Check sheet for the drawn part. Datum: minimum x, y, z corner. Units: mm. A direction names the side the tool comes from. Round coordinates to 2 decimals unless told otherwise and drop trailing zeros. Order: outer loops, then holes, each group sorted by start corner. A loop starts at its lowest first (then second) coordinate and runs counter-clockwise, first axis right, second up. Notation, with made-up numbers: (78.25, 35) -> (83.25, 35) arc R33 cw to (83.25, 69) -> close; hole circle Ø6 at (40.5, 19). An arc over 180 degrees is marked (long way). Write item = value, one per line. Start each with the question number.
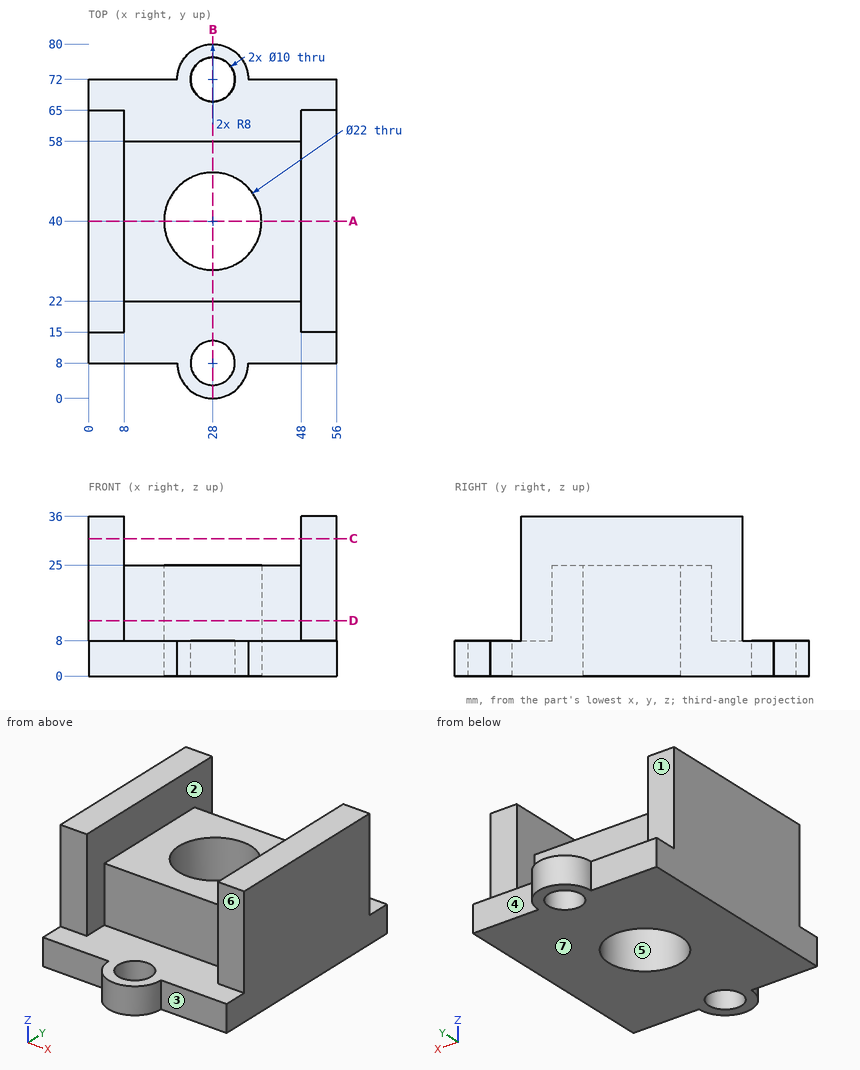
(1) Cross-section at B-B (x = 28). Enter the section's corners in (y, z), and give its area (3 significant figures).
(2) Depth check by flat-ended pin: pin 1 (9 mm diameter, centred on x = 51, z = 5.5, fed in from +Y); pin 2 (4 mm diameter, centred on x = 50, z = 25, fed in from +Y); pin 3 (14 mm diameter, centred on y = 39.5, z = 19, fed in from -X); pin 4 (1 mm diameter, centred on x = 16, y = 65, fed in from +Z). Enter the tip coordinate at first touch or a pass-through.
(3) Set-up check for the marked faces 1, 2, 3 and 4: record each of +Z, -Z, +X, -X, +Y, -Y from which the full face is reachable in a straight line by a thin tool's end or side.
(4) Cross-section at A-A (y = 40). Enter the section's corners in (x, z).
(5) Cross-section at C-C (z = 31). Enter the section's corners in (x, y), and give its area (3 significant figures).
(6) Scan lines: line 1 along Y through (x, z) = (28, 5); line 2 along X through (y, z) = (33, 33.5); line 3 along Y through (x, z) = (49.5, 34). Record each from-to range of solid material in increasing order. Write a range as from..to.
(7) Draft check along Y on the marked faces 5, 6 and 7. Enter one of: +Y half, -Y half, draft (parallel to the pull), parting line (faces both ways), or undercut.
(8) Cross-section at D-D (z = 12.5). Enter the section's corners in (x, y).
Outcome:
q1.outline = (0, 0) -> (3, 0) -> (3, 8) -> (0, 8) -> close; (13, 0) -> (29, 0) -> (29, 25) -> (22, 25) -> (22, 8) -> (13, 8) -> close; (51, 0) -> (67, 0) -> (67, 8) -> (58, 8) -> (58, 25) -> (51, 25) -> close; (77, 0) -> (80, 0) -> (80, 8) -> (77, 8) -> close
q1.area = 542 mm^2
q2.pin_1 = 72
q2.pin_2 = 65
q2.pin_3 = 0
q2.pin_4 = 8
q3.face_1 = +Z, +X, -X, +Y
q3.face_2 = +Z
q3.face_3 = +Z, -Z, +X, -Y
q3.face_4 = +Z, -Z, +X, +Y
q4.outline = (0, 0) -> (17, 0) -> (17, 25) -> (8, 25) -> (8, 36) -> (0, 36) -> close; (39, 0) -> (56, 0) -> (56, 36) -> (48, 36) -> (48, 25) -> (39, 25) -> close
q5.outline = (0, 15) -> (8, 15) -> (8, 65) -> (0, 65) -> close; (48, 15) -> (56, 15) -> (56, 65) -> (48, 65) -> close
q5.area = 800 mm^2
q6.line_1 = 0..3, 13..29, 51..67, 77..80
q6.line_2 = 0..8, 48..56
q6.line_3 = 15..65
q7.face_5 = undercut
q7.face_6 = -Y half
q7.face_7 = draft
q8.outline = (0, 15) -> (8, 15) -> (8, 22) -> (48, 22) -> (48, 15) -> (56, 15) -> (56, 65) -> (48, 65) -> (48, 58) -> (8, 58) -> (8, 65) -> (0, 65) -> close; hole circle Ø22 at (28, 40)
